```python
from build123d import *

# Parameters (mm, degrees)
FASE1_SIZE                                           = 1
FASE2_SIZE                                           = 1
FORMSENKUNG_F_R_M3_SENKSCHRAUBE_MIT_SCHL_D           = 3.4
FORMSENKUNG_F_R_M3_SENKSCHRAUBE_MIT_SCHL_CSINK_D     = 6.3
FORMSENKUNG_F_R_M3_SENKSCHRAUBE_MIT_SCHL_CSINK_ANGLE = 90
KREISMUSTER1_COUNT                                   = 6


with BuildPart() as part:
    # Skizze1 → Rotation1 (revolve)
    with BuildSketch(Plane.XY, mode=Mode.PRIVATE) as rotation1_sk:
        Polygon((10.25, 0), (20, 0), (20, 7), (32.5, 7), (32.5, 13), (16, 13), (16, 6), (10.25, 6), align=None)
    revolve(rotation1_sk.sketch.rotate(Axis((0, 0, 0), (0, -1, 0)), 90), axis=Axis((0, 0, 0), (0, -1, 0)))

    # Fase1
    fase1_edges = [part.edges().sort_by_distance(p)[0] for p in [
        (0, 13, -16),
    ]]
    chamfer(fase1_edges, length=FASE1_SIZE)

    # Fase2
    fase2_edges = [part.edges().sort_by_distance(p)[0] for p in [
        (0, 0, -20),
    ]]
    chamfer(fase2_edges, length=FASE2_SIZE)

    # Formsenkung für M3 Senkschraube mit Schlitz/Kreuzschlitz1 (through all)
    with Locations(Plane(origin=(0, 7, 0), x_dir=(-1, 0, 0), z_dir=(0, -1, 0))):
        with Locations((0, 25)):
            formsenkung_f_r_m3_senkschraube_mit_schl = CounterSinkHole(FORMSENKUNG_F_R_M3_SENKSCHRAUBE_MIT_SCHL_D / 2, FORMSENKUNG_F_R_M3_SENKSCHRAUBE_MIT_SCHL_CSINK_D / 2, counter_sink_angle=FORMSENKUNG_F_R_M3_SENKSCHRAUBE_MIT_SCHL_CSINK_ANGLE)

    # Kreismuster1: Formsenkung für M3 Senkschraube mit Schlitz/Kreuzschlitz1 ×6 about axis
    kreismuster1_axis = Axis((0, 0, 0), (0, 1, 0))
    for i in range(1, KREISMUSTER1_COUNT):
        add(formsenkung_f_r_m3_senkschraube_mit_schl.rotate(kreismuster1_axis, i * 360 / KREISMUSTER1_COUNT), mode=Mode.SUBTRACT)


solid = part.part
```
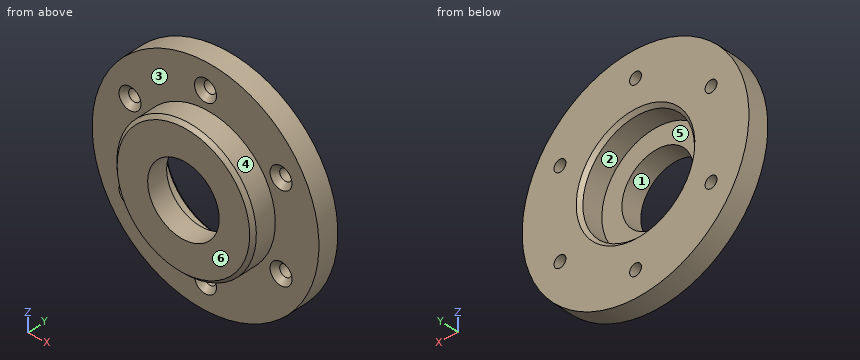
Work out the finished part from the listing and answer in its coordinate system (mm). Face numbers are marked on the shaded views. A direction names the side the tool comes from. Give positions to 0.01 mm unless a question says otherwise; leave off trailing zeros. Order: outer loops, then holes, each group sorted by start corner. A loop starts at its lowest first (then second) coordinate and runs counter-clockwise, first axis right, second up.
1. Section B-B, the plane y = 2 is taken. Determine the outline of the cut face in (x, z).
Result sheet:
outline: circle Ø40 at (0, 0); hole circle Ø20.5 at (0, 0)
2. Section C-C, the plane y = 11.25 is taken. Determine the outline of the cut face in (x, z).
Result sheet:
outline: circle Ø65 at (0, 0); hole circle Ø3.4 at (-21.65, -12.5); hole circle Ø3.4 at (-21.65, 12.5); hole circle Ø32 at (0, 0); hole circle Ø3.4 at (0, -25); hole circle Ø3.4 at (0, 25); hole circle Ø3.4 at (21.65, -12.5); hole circle Ø3.4 at (21.65, 12.5)
3. The mould has two halves that part along Z. Classify the marked faces 4, 5 and 6: released by +Z, released by -Z, zero draft, split by the parting line, or undercut.
Result sheet:
face 4: split by the parting line
face 5: undercut
face 6: zero draft
4. For the marked faces 1, 2 and 3, determine the directions among +Z, -Z, +X, -X, +Y, -Y from which every point of the face is accessible in a straight line to the end or side of a thin tool.
Result sheet:
face 1: +Y, -Y
face 2: +Y
face 3: -Y
5. Each of these flat-tipped pins is pushed along its axis until it touches: P1, Ø4.5, axis at x = -21.65, z = 12.5, coming from the -Y side; P2, Ø1.5, axis at y = 9.5, z = 8.5, coming from the +X side; P3, Ø5, axis at x = -2.5, y = 4, coming from the -Z side. Where does it stop, or does it pass through?
Result sheet:
P1: stops at y = 7.9
P2: stops at x = 31.56
P3: stops at z = -20
6. Section D-D, the plane z = -25 is taken. Determine the outline of the cut face in (x, y), and give its area (3 significant figures).
Result sheet:
outline: (-20.77, 7) - (-3.15, 7) - (-1.7, 8.45) - (-1.7, 13) - (-20.77, 13) - close; (1.7, 8.45) - (3.15, 7) - (20.77, 7) - (20.77, 13) - (1.7, 13) - close
area: 227 mm2
7. Section A-A, the plane z = 0 is taken. Determine the outline of the cut face in (x, y), and give its area (3 significant figures).
Result sheet:
outline: (-32.5, 7) - (-20, 7) - (-20, 1) - (-19, 0) - (-10.25, 0) - (-10.25, 6) - (-16, 6) - (-16, 12) - (-17, 13) - (-32.5, 13) - close; (10.25, 0) - (19, 0) - (20, 1) - (20, 7) - (32.5, 7) - (32.5, 13) - (17, 13) - (16, 12) - (16, 6) - (10.25, 6) - close
area: 321 mm2
8. Straight lines are drawn through the part: L1, parallel to X at y = 10.7, z = 0; L2, parallel to X at y = 11.25, z = -14; L3, parallel to X at y = 10.6, z = -12.5. For each, find the intervals that lie inside material, in ascending order.
Result sheet:
L1: x = -32.5 to -16, 16 to 32.5
L2: x = -29.33 to -22.45, -20.85 to -7.75, 7.75 to 20.85, 22.45 to 29.33
L3: x = -30 to -23.35, -19.95 to -9.99, 9.99 to 19.95, 23.35 to 30
